from build123d import *

# Parameters (mm, degrees)
CHAMFER1_SIZE = 0.1125
CHAMFER2_SIZE = 0.0375
FILLET1_R     = 0.06


with BuildPart() as part:
    # Sketch3 → Revolve1 (revolve)
    with BuildSketch(Plane(origin=(0, 0, 0), x_dir=(0, 0, -1), z_dir=(1, 0, 0)), mode=Mode.PRIVATE) as revolve1_sk:
        Polygon((1.5, -4.75), (0.75, -4.75), (0.75, -2.75), (-1.5, -2.75), (-1.5, -2), (1.5, -2), align=None)
    revolve(revolve1_sk.sketch.rotate(Axis((0, 0, 1.5), (0, 0, -1)), 270), axis=Axis((0, 0, 1.5), (0, 0, -1)))

    # Chamfer1
    chamfer1_edges = [part.edges().sort_by_distance(p)[0] for p in [
        (-2.75, 0, 1.5),
    ]]
    chamfer(chamfer1_edges, length=CHAMFER1_SIZE)

    # Chamfer2
    chamfer2_edges = [part.edges().sort_by_distance(p)[0] for p in [
        (-2, 0, -1.5),
        (-2, 0, 1.5),
    ]]
    chamfer(chamfer2_edges, length=CHAMFER2_SIZE)

    # Fillet1
    fillet1_edges = [part.edges().sort_by_distance(p)[0] for p in [
        (-2.75, 0, -0.75),
        (-4.75, 0, -0.75),
        (-4.75, 0, -1.5),
    ]]
    fillet(fillet1_edges, radius=FILLET1_R)


solid = part.part
Model file for the job. Use its own axes, mm. A direction names the side the tool comes from. Coordinates: 2 decimals unless noted, no trailing zeros. Write each loop counter-clockwise with the first axis right and the second up, starting at its lowest first coordinate (ties: lowest second). Pieces come first, ordered by that corner, then holes. Notation, with made-up numbers: (66, 35) -> (99, 35) arc R25 ccw to (99, 66) -> close; hole circle Ø9 at (82.5, 30). An arc over 180 degrees is marked (long way). One line per item, written item: value. Start each with the question number.
1) Slice it at A-A on y = 0. Write the cut outline in (x, z), then the cut area to 3 significant figures.
2) Slice it at C-C on z = 0.05. Write the cut outline in (x, y).
3) Probe probe 1 along Y at (x, z) = (0, -0.35); probe 2 along Z at (x, y) = (-2, 3.5); probe 3 along Y at (x, z) = (-1.25, 0.1). List the from-to ranges inside material, lowest first.
4) Pull direction X, two halves, no side cores. Call faces 1 (the face through (0, 2, 0)), 2 (the face through (0, 3, -0.75)), 3 (the face through (-3.77, 2.89, -1.12)): +X half, -X half, draft (parallel to the pull), parting line (faces both ways), or undercut.
5) Slice it at D-D on z = -1.1. Write the cut outline in (x, y).
6) Which spindle directions (+Z, -Z, +X, -X, +Y, -Y) get a long thin tool onto all of the face, cutting with end or side? Do faces 4 (the face through (-0.596, 2.685, 0.363)), 5 (the face through (-2, 1, -1.5)). Say none if no direction does.
Answers follow:
1. outline: (-4.75, -1.44) arc R0.06 ccw to (-4.69, -1.5) -> (-2.04, -1.5) -> (-2, -1.46) -> (-2, 1.46) -> (-2.04, 1.5) -> (-2.64, 1.5) -> (-2.75, 1.39) -> (-2.75, -0.69) arc R0.06 cw to (-2.81, -0.75) -> (-4.69, -0.75) arc R0.06 ccw to (-4.75, -0.81) -> close; (2, -1.46) -> (2.04, -1.5) -> (4.69, -1.5) arc R0.06 ccw to (4.75, -1.44) -> (4.75, -0.81) arc R0.06 ccw to (4.69, -0.75) -> (2.81, -0.75) arc R0.06 cw to (2.75, -0.69) -> (2.75, 1.39) -> (2.64, 1.5) -> (2.04, 1.5) -> (2, 1.46) -> close
1. area: 7.48 mm2
2. outline: circle Ø5.5 at (0, 0); hole circle Ø4 at (0, 0)
3. probe 1: -2.75 to -2, 2 to 2.75
3. probe 2: -1.5 to -0.75
3. probe 3: -2.45 to -1.56, 1.56 to 2.45
4. face 1: undercut
4. face 2: draft
4. face 3: parting line
5. outline: circle Ø9.5 at (0, 0); hole circle Ø4 at (0, 0)
6. face 4: +Z
6. face 5: -Z, +X, -X, +Y, -Y
